Model file for the job. Use its own axes, mm. A direction names the side the tool comes from. Coordinates: 2 decimals unless noted, no trailing zeros. Order: outer loops, then holes, each group sorted by start corner. A loop starts at its lowest first (then second) coordinate and runs counter-clockwise, first axis right, second up.
Autodesk Inventor part; units mm, degrees
ref_plane "YZ Plane" through (0, 0, 0) normal (1, 0, 0) x (0, 1, 0)
ref_plane "XZ Plane" through (0, 0, 0) normal (0, 1, 0) x (-1, 0, 0)
ref_plane "XY Plane" through (0, 0, 0) normal (0, 0, 1) x (1, 0, 0)
sketch "Sketch1" plane through (0, 0, 0) normal (0, 1, 0) x (-1, 0, 0)
  line L0 (-12.7, -12.7) -> (12.7, -12.7)
  line L1 (12.7, -12.7) -> (12.7, 12.7)
  line L2 (12.7, 12.7) -> (-12.7, 12.7)
  line L3 (-12.7, 12.7) -> (-12.7, -12.7)
  line L4 (-12.7, -12.7) -> (12.7, 12.7) construction
  line L5 (12.7, -12.7) -> (-12.7, 12.7) construction
  line L6 (9.525, 9.525) -> (9.525, -9.525)
  line L7 (9.525, -9.525) -> (-9.525, -9.525)
  line L8 (-9.525, -9.525) -> (-9.525, 9.525)
  line L9 (-9.525, 9.525) -> (9.525, 9.525)
  point P0 (0, 0)
  dimension "d0" = 25.4
  dimension "d1" = 25.4
  dimension "d2" = 3.175
extrude "Extrusion1" add sketch "Sketch1" along normal mid plane 711.2
sketch "Sketch2" plane through (-12.7, 355.6, 12.7) normal (0, 0, 1) x (1, 0, 0)
  line L0 (0, 0) -> (25.4, 0)
  line L1 (0, 0) -> (25.4, -25.4)
  line L2 (25.4, -711.2) -> (25.4, 0)
  circle A0 centre (12.7, -31.75) radius 3.2512
  circle A1 centre (12.7, -50.8) radius 3.2512
  line L3 (0, -711.2) -> (0, 0)
  line L4 (0, -355.6) -> (25.4, -355.6) construction
  line L5 (0, -711.2) -> (25.4, -711.2)
  line L6 (0, -711.2) -> (25.4, -685.8)
  circle A2 centre (12.7, -679.45) radius 3.2512
  circle A3 centre (12.7, -660.4) radius 3.2512
  circle A4 centre (12.7, -12.7) radius 3.2512
  circle A5 centre (12.7, -698.5) radius 3.2512
  point P0 (12.7, -355.6)
  point P1 (12.7, 0)
  point P2 (12.7, -711.2)
  point P3 (14.9989, -14.9989)
  point P4 (10.4011, -10.4011)
  point P5 (14.9989, -696.2011)
  point P6 (10.4011, -700.7989)
  dimension "d5" = 25.4
  dimension "d6" = 6.5024
  dimension "d7" = 31.75
  dimension "d8" = 19.05
extrude "Extrusion2" cut sketch "Sketch2" against normal blind 711.2 contours L0 L2 L1 A4 | A4 L1 | L1 A4 | L6 A5 L2 L5 | A5 L6 | L6 A5 | A0 | A1 | A2 | A3
sketch "Sketch3" plane through (-12.7, -355.6, 12.7) normal (0, 0, 1) x (1, 0, 0)
  line L0 (0, 711.2) -> (0, 0) construction
  line L1 (0, 355.6) -> (25.4, 355.6) construction
  line L2 (25.4, 25.4) -> (25.4, 685.8) construction
  circle A0 centre (12.7, 171.45) radius 3.2512
  circle A1 centre (12.7, 539.75) radius 3.2512
  point P0 (12.7, 355.6)
  dimension "d14" = 6.5024
  dimension "d15" = 184.15
  dimension "d16" = 146.05
extrude "Extrusion3" cut sketch "Sketch3" against normal blind 25.4
properties part number "STRU_003_BilletPole_28in_Angled" material "Aluminum 6061"
Q1. Probe line 1 (X direction, y = 5, z = -4.5) (3 decimals); line 2 (X direction, y = 304.8, z = -12). List the from-to ranges inside material, lowest first.
Established:
line 1: x = -12.7 to -9.525, 9.525 to 12.7
line 2: x = -12.7 to -3.25, 3.25 to 12.7
Q2. Mould opens along Z. For faces 1 (the face through (0, -5, -12.7)), 2 (the face through (12.7, -5, 0)), 3 (the face through (0, -5, 9.525)), 4 (the face through (9.525, -5, 0)) say: pulls with the +Z half, pulls with the -Z half, needs draft (parallel to the pull), parting line crosses it, or undercut.
Established:
face 1: pulls with the -Z half
face 2: needs draft
face 3: undercut
face 4: undercut
Q3. Cut at B-B, the plane y = -28. List the corners of the cut face in (x, z) (3 decimals).
Established:
outline: (-12.7, -12.7) - (12.7, -12.7) - (12.7, 12.7) - (-12.7, 12.7) - close; hole (-9.525, -9.525) - (9.525, -9.525) - (9.525, 9.525) - (-9.525, 9.525) - close
Q4. Which spindle directions (+Z, -Z, +X, -X, +Y, -Y) get a long thin tool onto all of the face, cutting with end or side? Do faces 5 (the face through (0, -5, -9.525)), 6 (the face through (0, -5, 12.7)). Say none if no direction does.
Established:
face 5: +Y, -Y
face 6: +Z, +X, -X, +Y, -Y
Q5. Cut at A-A, the plane z = -5.25. List the corners of the cut face in (x, y) (3 decimals).
Established:
outline: (-12.7, -355.6) - (-9.525, -352.425) - (-9.525, 352.425) - (-12.7, 355.6) - close; (9.525, -333.375) - (12.7, -330.2) - (12.7, 330.2) - (9.525, 333.375) - close
